Autodesk Fusion 360 part; units mm, degrees
sketch "Sketch1" plane through (0, 0, 0) normal (0, 0, 1) x (1, 0, 0)
  line L0 (-100, 0) -> (100, 0)
  line L1 (100, 0) -> (91.75, 0) construction
  line L2 (91.75, 0) -> (91.75, 8.25) construction
  line L3 (91.75, 8.25) -> (100, 8.25) construction
  line L4 (100, 8.25) -> (100, 0) construction
  line L5 (-100, 0) -> (-91.75, 0) construction
  line L6 (-91.75, 0) -> (-91.75, 8.25) construction
  line L7 (-91.75, 8.25) -> (-100, 8.25) construction
  line L8 (-100, 8.25) -> (-100, 0) construction
  circle A0 centre (-91.75, 8.25) radius 3.25
  circle A1 centre (91.75, 8.25) radius 3.25
  line L9 (0, 0) -> (0, 60) construction
  line L10 (-48.5, 60) -> (48.5, 60) construction
  line L11 (48.5, 85) -> (60.5, 85) construction
  line L12 (60.5, 85) -> (60.5, 35) construction
  line L13 (60.5, 35) -> (48.5, 35) construction
  line L14 (48.5, 35) -> (48.5, 85) construction
  line L15 (-60.5, 85) -> (-48.5, 85) construction
  line L16 (-48.5, 85) -> (-48.5, 35) construction
  line L17 (-48.5, 35) -> (-60.5, 35) construction
  line L18 (-60.5, 35) -> (-60.5, 85) construction
  line L19 (0, 0) -> (0, 8.25) construction
  line L20 (22.5, 8.25) -> (22.5, 78.25) construction
  line L21 (22.5, 78.25) -> (-22.5, 78.25) construction
  line L22 (-22.5, 78.25) -> (-22.5, 8.25) construction
  circle A2 centre (-22.5, 78.25) radius 3.25
  circle A3 centre (22.5, 78.25) radius 3.25
  circle A4 centre (22.5, 8.25) radius 3.25
  circle A5 centre (-22.5, 8.25) radius 3.25
  line L23 (-48.5, 35) -> (-55.5711, 27.9289) construction
  line L24 (-60.5, 35) -> (-53.4289, 27.9289) construction
  line L25 (-60.5, 35) -> (-48.5, 35) construction
  line L26 (48.5, 35) -> (55.5711, 27.9289) construction
  line L27 (48.5, 35) -> (60.5, 35) construction
  line L28 (60.5, 35) -> (53.4289, 27.9289) construction
  line L29 (-54.5, 29) -> (-38.9437, 44.5563) construction
  line L30 (-54.5, 29) -> (-70.0563, 44.5563) construction
  line L31 (54.5, 29) -> (70.0563, 44.5563) construction
  line L32 (54.5, 29) -> (38.9437, 44.5563) construction
  line L33 (22.5, 8.25) -> (-22.5, 8.25) construction
  line L34 (70.0563, 44.5563) -> (72.1777, 42.435) construction
  line L35 (38.9437, 44.5563) -> (36.8223, 42.435) construction
  line L36 (-38.9437, 44.5563) -> (-36.8223, 42.435) construction
  line L37 (-70.0563, 44.5563) -> (-72.1777, 42.435) construction
  line L38 (72.1777, 42.435) -> (54.5, 24.7574)
  line L39 (36.8223, 42.435) -> (54.5, 24.7574)
  line L40 (-36.8223, 42.435) -> (-54.5, 24.7574)
  line L41 (-72.1777, 42.435) -> (-54.5, 24.7574)
  line L42 (-36.8223, 42.435) -> (-36.8223, 86.5)
  line L43 (36.8223, 42.435) -> (36.8223, 86.5)
  line L44 (36.8223, 86.5) -> (-36.8223, 86.5)
  line L45 (45.6612, 33.5962) -> (40.3579, 28.2929) construction
  line L46 (-45.6612, 33.5962) -> (-40.3579, 28.2929) construction
  line L47 (-40.3579, 28.2929) -> (-36.8223, 31.8284)
  line L48 (-36.8223, 31.8284) -> (-33.2868, 28.2929)
  line L49 (-33.2868, 28.2929) -> (-40.3579, 21.2218)
  line L50 (-40.3579, 21.2218) -> (-43.8934, 24.7574)
  line L51 (-43.8934, 24.7574) -> (-40.3579, 28.2929)
  line L52 (40.3579, 28.2929) -> (36.8223, 31.8284)
  line L53 (36.8223, 31.8284) -> (33.2868, 28.2929)
  line L54 (33.2868, 28.2929) -> (40.3579, 21.2218)
  line L55 (40.3579, 21.2218) -> (43.8934, 24.7574)
  line L56 (43.8934, 24.7574) -> (40.3579, 28.2929)
  line L57 (-91.75, 8.25) -> (-91.75, 16.5) construction
  line L58 (91.75, 8.25) -> (91.75, 16.5) construction
  line L59 (100, 16.5) -> (100, 0)
  line L60 (-100, 16.5) -> (-100, 0)
  line L61 (72.1777, 42.435) -> (100, 16.5)
  line L62 (-72.1777, 42.435) -> (-100, 16.5)
  line L63 (-36.8223, 42.435) -> (-31.519, 37.1317)
  line L64 (-31.519, 37.1317) -> (-49.1967, 19.4541)
  line L65 (-49.1967, 19.4541) -> (-54.5, 24.7574)
  line L66 (36.8223, 42.435) -> (31.519, 37.1317)
  line L67 (31.519, 37.1317) -> (49.1967, 19.4541)
  line L68 (49.1967, 19.4541) -> (54.5, 24.7574)
  line L69 (36.8223, 42.435) -> (36.8223, 31.8284)
  circle A6 centre (0, 8.25) radius 3.25
  circle A7 centre (0, 78.25) radius 3.25
  line L70 (-35, 43.25) -> (-10, 43.25) construction
  line L71 (-35, 40.6127) -> (-35, 33.6508)
  line L72 (10, 43.25) -> (35, 43.25) construction
  line L73 (35, 40.6127) -> (35, 33.6508)
  dimension "d2" = 200
  dimension "d3" = 8.25
  dimension "d4" = 8.25
  dimension "d5" = 8.25
  dimension "d6" = 8.25
  dimension "d7" = 6.5
  dimension "d8" = 6.5
  dimension "d9" = 60
  dimension "d10" = 97
  dimension "d11" = 12
  dimension "d12" = 50
  dimension "d13" = 12
  dimension "d14" = 50
  dimension "d15" = 8.25
  dimension "d16" = 45
  dimension "d17" = 70
  dimension "d18" = 6.5
  dimension "d19" = 6.5
  dimension "d20" = 6.5
  dimension "d21" = 6.5
  dimension "d22" = 10
  dimension "d24" = 45
  dimension "d25" = 10
  dimension "d26" = 45
  dimension "d27" = 10
  dimension "d28" = 10
  dimension "d29" = 22
  dimension "d30" = 22
  dimension "d31" = 22
  dimension "d32" = 22
  dimension "d33" = 3
  dimension "d34" = 3
  dimension "d35" = 3
  dimension "d36" = 3
  dimension "d37" = 25
  dimension "d38" = 25
  dimension "d39" = 25
  dimension "d41" = 25
  dimension "d44" = 7.5
  dimension "d45" = 7.5
  dimension "d46" = 5
  dimension "d47" = 5
  dimension "d48" = 10
  dimension "d49" = 5
  dimension "d50" = 5
  dimension "d51" = 5
  dimension "d52" = 10
  dimension "d53" = 5
  dimension "d54" = 86.5
  dimension "d57" = 8.25
  dimension "d58" = 8.25
  dimension "d69" = 7.5
  dimension "d70" = 25
  dimension "d71" = 7.5
  dimension "d72" = 25
  dimension "d85" = 6.5
  dimension "d86" = 6.5
  dimension "d87" = 25
  dimension "d88" = 25
extrude "Extrude2" add sketch "Sketch1" along normal blind 10 contours L0 L38 L41 L42 L43 L44 L48 L49 L50 L53 L54 L55 L59 L60 L61 L62 L63 L64 L65 L66 L67 L68 | L40 L47 L51 L63 L64 L65 L71 | L66 L67 L69 L73 | L63 L64 L71 | L47 L48 L49 L50 L51 L64 | L66 L67 L73 | L52 L53 L54 L55 L56 L67
extrude "Extrude3" add sketch "Sketch1" along normal blind 27.45 contours L40 L47 L51 L63 L64 L65 L71 | L39 L52 L56 L67 L68 L69 | L66 L67 L69 L73
sketch "Sketch4" plane through (39.6287, 39.6287, 0) normal (0.7071, 0.7071, 0) x (-0.7071, 0.7071, 0)
  line L0 (-21.0312, 0) -> (3.9688, 0)
  line L1 (3.9688, 27.45) -> (-21.0312, 27.45)
  line L2 (-21.0312, 27.45) -> (-21.0312, 10)
  line L3 (-21.0312, 10) -> (-21.0312, 0)
  line L4 (-8.5312, 27.45) -> (-8.5312, 19.2) construction
  line L5 (3.9688, 0) -> (3.9688, 10)
  line L6 (3.9688, 10) -> (3.9688, 27.45)
  dimension "d77" = 8.25
sketch "Sketch5" plane through (-39.6287, 39.6287, 0) normal (-0.7071, 0.7071, 0) x (-0.7071, -0.7071, 0)
  line L0 (-3.9688, 0) -> (21.0312, 0)
  line L1 (21.0312, 0) -> (21.0312, 10)
  line L2 (21.0312, 10) -> (21.0312, 27.45)
  line L3 (21.0312, 27.45) -> (-3.9688, 27.45)
  line L4 (8.5312, 27.45) -> (8.5312, 19.2) construction
  line L5 (-3.9688, 10) -> (-3.9688, 0)
  line L6 (-3.9688, 27.45) -> (-3.9688, 10)
  dimension "d78" = 8.25
hole "Hole3" at (-45.6612, 33.5962, 19.2) direction (0.7071, -0.7071, 0) diameter 6.5 depth 7.5 tip angle 180
hole "Hole4" at (45.6612, 33.5962, 19.2) direction (-0.7071, -0.7071, 0) diameter 6.5 depth 7.5 tip angle 180
equation "d3 = 5 mm + 3.25 mm"
equation "d4 = 5 mm + 3.25 mm"
equation "d5 = 5 mm + 3.25 mm"
equation "d6 = 5 mm + 3.25 mm"
equation "d10 = 121 mm - 24 mm"
equation "d15 = 5 mm + 3.25 mm"
equation "d54 = 90 mm - 3.5 mm"
equation "d75 = 30.7 mm - 3.25 mm"
Design review of the part built by this model. Coordinates are the model's own, in mm. A direction names the side the tool comes from. Give positions to 0.01 mm unless a question says otherwise; leave off trailing zeros. Order: outer loops, then holes, each group sorted by start corner. A loop starts at its lowest first (then second) coordinate and runs counter-clockwise, first axis right, second up. Notation, with made-up numbers: (-15, -8) -> (11, -8) arc R11 cw to (11, 1) -> close; hole circle Ø8 at (1, 4.5). An arc over 180 degrees is marked (long way). Write each question's results on one line, items separated by ' | '. Start each with the question number.
Q1. Add section A-A on y = 78.25. Give the boundary of the cut face in (x, z), and give its area (3 significant figures).
Q2. For pin 1 (2 mm diameter, centred on x = 14.5, y = 32.5, fed in from +Z); pin 2 (3.5 mm diameter, centred on y = 38.5, z = 19.5, fed in from -X); pin 3 (2 mm diameter, centred on x = 46.5, z = 18, fed in from +Y), all flat-tipped, find the tip position at first contact; note any pin that passes through.
Q3. Add section C-C on z = 6.75. State how many separate pieces and enclosed holes the cut face has, and give its area (3 significant figures).
Q4. Mouldability with a two-part tool opening along Z and no side actions: class faces 5 (the cylindrical face through (42.871, 31.008, 15.953)), 6 (the cylindrical face through (-25.1, 80.2, 4.9)), 7 (the flat face through (-1, 34, 0)) as +Z half, -Z half, draft (parallel to the pull), parting line (faces both ways), or undercut.
Q5. Add section B-B on x = 0. Give the boundary of the cut face in (y, z).
Q6. Wall thickness on L1, parallel to Y at x = 22.5, z = 7.25; L2, parallel to X at y = 78, z = 6; L3, parallel to X at y = 30.5, z = 12: over which ranges is each line inside the solid? List them lowest first. Write a range as from..to.
Q7. Add section D-D on x = 91.75. Give the boundary of the cut face in (y, z).
Q8. Machinability: for faces 1 (the flat face through (-51.81, 22.07, 18.6)), 2 (the flat face through (35, 37, 19)), 3 (the flat face through (51.81, 22.07, 18.6)), 4 (the flat face through (45.54, 33.72, 13.53)), which of the approach directions +Z, -Z, +X, -X, +Y, -Y give a long, thin tool a straight path to every point of the face, cutting with its end or side? Answer none if there is none.
Found:
1) outline: (-36.82, 0) -> (-25.75, 0) -> (-25.75, 10) -> (-36.82, 10) -> close; (-19.25, 0) -> (-3.25, 0) -> (-3.25, 10) -> (-19.25, 10) -> close; (3.25, 0) -> (19.25, 0) -> (19.25, 10) -> (3.25, 10) -> close; (25.75, 0) -> (36.82, 0) -> (36.82, 10) -> (25.75, 10) -> close | area: 541 mm2
2) pin 1: stops at z = 10 | pin 2: stops at x = -42.51 | pin 3: stops at y = 31.42
3) separate pieces: 1 | enclosed holes: 8 | area: 10,100 mm2
4) face 5: undercut | face 6: draft | face 7: -Z half
5) outline: (0, 0) -> (5, 0) -> (5, 10) -> (0, 10) -> close; (11.5, 0) -> (75, 0) -> (75, 10) -> (11.5, 10) -> close; (81.5, 0) -> (86.5, 0) -> (86.5, 10) -> (81.5, 10) -> close
6) L1: y = 0..5, 11.5..75, 81.5..86.5 | L2: x = -36.82..-25.74, -19.26..-3.24, 3.24..19.26, 25.74..36.82 | L3: x = -48.76..-38.15, 38.15..48.76
7) outline: (0, 0) -> (5, 0) -> (5, 10) -> (0, 10) -> close; (11.5, 0) -> (24.19, 0) -> (24.19, 10) -> (11.5, 10) -> close
8) face 1: +Z, -X, -Y | face 2: +Z, +Y, -Y | face 3: +Z, +X, -Y | face 4: +Z, -Z, +Y
